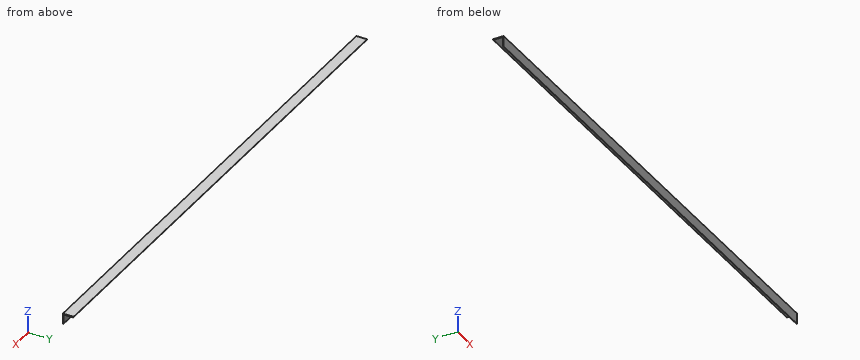
```python
from build123d import *

# Parameters (mm, degrees)
L_ANGLE_EQUAL_40X40X3_2_DEPTH = 1920


with BuildPart() as part:
    # Sketch13 → L angle (equal) 40X40X3(2) (new body)
    with BuildSketch(Plane(origin=(0, 0, 0), x_dir=(0, 0, -1), z_dir=(1, 0, 0))):
        with BuildLine():
            Line((0, 40), (0, 0))
            Line((0, 0), (40, 0))
            ThreePointArc((40, 0), (39.121320344, 2.121320344), (37, 3))
            Line((37, 3), (9, 3))
            ThreePointArc((9, 3), (4.757359313, 4.757359313), (3, 9))
            Line((3, 9), (3, 37))
            ThreePointArc((3, 37), (2.121320344, 39.121320344), (0, 40))
        make_face()
    extrude(amount=L_ANGLE_EQUAL_40X40X3_2_DEPTH)


solid = part.part
```
Here's how the part is built. I have some questions about the finished solid (model axes, mm). Round coordinates to 2 decimals unless told otherwise and drop trailing zeros. Order: outer loops, then holes, each group sorted by start corner. A loop starts at its lowest first (then second) coordinate and runs counter-clockwise, first axis right, second up. Notation, with made-up numbers: M -29,83.25 L 15,83.25 A36 cw 15,119.25 Z; hole C -36,-19.75 d8. An arc over 180 degrees is marked long. One line per question, with ' | ' between items.
1) I want a section at C-C, the plane z = -20.5. Write out the boundary of the cut face in (x, y).
Working result:
outline: M 0,0 L 1920,0 L 1920,3 L 0,3 Z
2) I need wall thicknesses on line 1 along Z through (x, y) = (1831, 27); line 2 along Y through (x, z) = (921, -16); line 3 along Z through (x, y) = (1500, 7). Which ranges of each line are inside material? Lowest first, please.
Working result:
line 1: -3 to 0 | line 2: 0 to 3 | line 3: -3.34 to 0
3) I want a section at A-A, the plane x = 857.5. Write out the boundary of the cut face in (y, z), then the cut area to 3 significant figures.
Working result:
outline: M 0,-40 A3 ccw 3,-37 L 3,-9 A6 cw 9,-3 L 37,-3 A3 ccw 40,0 L 0,0 Z | area: 235 mm²
4) I want a section at B-B, the plane y = 30.5. Write out the boundary of the cut face in (x, z), then the cut area to 3 significant figures.
Working result:
outline: M 0,-3 L 1920,-3 L 1920,0 L 0,0 Z | area: 5,760 mm²
5) For pin 1 Ø3 at (x, z) = (830, -10) entering from -Y; pin 2 Ø8 at (x, y) = (1487, 34.5) entering from -Z; pin 3 Ø22.5 at (x, y) = (1433, 16.5) entering from -Z; pin 4 Ø12 at (y, z) = (23, -12) entering from -X, each with a flat end and sliding along its axis, tell me the tip position at first contact or that it passes through.
Working result:
pin 1: y = 0 | pin 2: z = -3 | pin 3: z = -4.32 | pin 4: through
